Geometry: final body of the model. Coordinates: model frame, mm. Round coordinates to 2 decimals unless told otherwise and drop trailing zeros. Loops run counter-clockwise (first coordinate to the right, second up) from the corner with the lowest first, then second, coordinate; pieces in that order, holes last. Notation, with made-up numbers: (-18.75, 25.25) - (9.25, 25.25) arc R18 ccw to (9.25, 51.25) - close; hole circle Ø7 at (71.25, -12). An arc over 180 degrees is marked (long way). Return JSON: item names as keys, results as strings. Group by question number.
1. Section A-A on x = 0. Return loops of the section in (y, z), and give its area (3 significant figures).
2. Section B-B on y = -33.25. Return loops of the section in (x, z), and give its area (3 significant figures).
3. Section C-C on x = 84. Return loops of the section in (y, z).
4. First-contact query: pin 1 Ø5.5 at (x, y) = (-57.59, 33.25) entering from +Z. Flat tip, straight axial feed; report the tip coordinate or a pass-through.
5. Section D-D on z = 1.6. Count the separate pieces of the cut face and the enclosed holes in it, and give its area (3 significant figures).
6. Material intervals for probe 1 along Y at (x, z) = (47, 1.55); probe 2 along Y at (x, z) = (1, 2.45); probe 3 along X at (y, z) = (4, 1.3), sorted ascending.
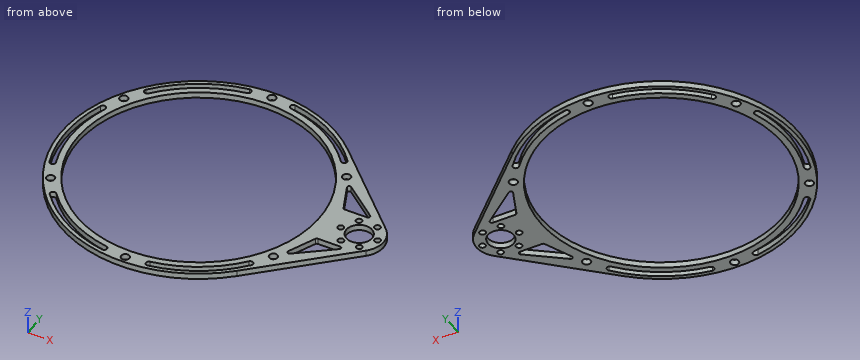
from build123d import *

# Parameters (mm, degrees)
SKETCH_1_R          = 2.1
SKETCH_1_R_2        = 61.75
SKETCH_1_R_3        = 1.55
SKETCH_1_R_4        = 6.6
EXTRUDE_1_DEPTH     = 3
CUT_EXTRUDE_1_DEPTH = 119.445134978
FILLET_1_R          = 1
CUT_EXTRUDE_2_DEPTH = 119.445134978


with BuildPart() as part:
    # 草图1 → 凸台-拉伸1 (new body)
    with BuildSketch(Plane.XY):
        with BuildLine():
            Line((91.659638554, 9.014469486), (48.493975904, 50.48102912))
            ThreePointArc((48.493975904, 50.48102912), (-70, 0), (48.493975904, -50.48102912))
            Line((48.493975904, -50.48102912), (91.659638554, -9.014469486))
            ThreePointArc((91.659638554, -9.014469486), (95.5, 0), (91.659638554, 9.014469486))
        make_face()
        with Locations((0, 66.5)):
            Circle(SKETCH_1_R, mode=Mode.SUBTRACT)
        with Locations((57.590689352, 33.25)):
            Circle(SKETCH_1_R, mode=Mode.SUBTRACT)
        with Locations((0, -66.5)):
            Circle(SKETCH_1_R, mode=Mode.SUBTRACT)
        with Locations((-57.590689352, -33.25)):
            Circle(SKETCH_1_R, mode=Mode.SUBTRACT)
        with Locations((57.590689352, -33.25)):
            Circle(SKETCH_1_R, mode=Mode.SUBTRACT)
        with Locations((-57.590689352, 33.25)):
            Circle(SKETCH_1_R, mode=Mode.SUBTRACT)
        Circle(SKETCH_1_R_2, mode=Mode.SUBTRACT)
        with Locations((87.75, 8.227241336)):
            Circle(SKETCH_1_R_3, mode=Mode.SUBTRACT)
        with Locations((78.25, -8.227241336)):
            Circle(SKETCH_1_R_3, mode=Mode.SUBTRACT)
        with Locations((87.75, -8.227241336)):
            Circle(SKETCH_1_R_3, mode=Mode.SUBTRACT)
        with Locations((73.5, 0)):
            Circle(SKETCH_1_R_3, mode=Mode.SUBTRACT)
        with Locations((83, 0)):
            Circle(SKETCH_1_R_4, mode=Mode.SUBTRACT)
        with Locations((78.25, 8.227241336)):
            Circle(SKETCH_1_R_3, mode=Mode.SUBTRACT)
        with Locations((92.5, 0)):
            Circle(SKETCH_1_R_3, mode=Mode.SUBTRACT)
    extrude(amount=EXTRUDE_1_DEPTH)

    # 草图2 → 切除-拉伸1 (cut, through all)
    with BuildSketch(Plane.XY.offset(3)):
        Polygon((59.859164826, 30.33893107), (67.889886949, 12.18949907), (83, 12.18949907), align=None)
        Polygon((67.889886949, -12.18949907), (83, -12.18949907), (59.859164826, -30.33893107), align=None)
    extrude(amount=-CUT_EXTRUDE_1_DEPTH, mode=Mode.SUBTRACT)

    # 圆角1
    fillet_1_edges = [part.edges().sort_by_distance(p)[0] for p in [
        (59.859164826, 30.33893107, 1.5),
        (83, 12.18949907, 1.5),
        (67.889886949, 12.18949907, 1.5),
        (59.859164826, -30.33893107, 1.5),
        (67.889886949, -12.18949907, 1.5),
        (83, -12.18949907, 1.5),
    ]]
    fillet(fillet_1_edges, radius=FILLET_1_R)

    # 草图3 → 切除-拉伸2 (cut, through all)
    with BuildSketch(Plane.XY.offset(3)):
        with BuildLine():
            ThreePointArc((52.091022132, 43.709557459), (34, 58.889727457), (11.808076081, 66.966927205))
            ThreePointArc((11.808076081, 66.966927205), (10.070392185, 65.750187842), (11.287131548, 64.012503946))
            ThreePointArc((11.287131548, 64.012503946), (32.5, 56.291651246), (49.792888803, 41.78119463))
            ThreePointArc((49.792888803, 41.78119463), (51.906136882, 41.596309379), (52.091022132, 43.709557459))
        make_face()
        with BuildLine():
            ThreePointArc((11.287131548, -64.012503946), (32.5, -56.291651246), (49.792888803, -41.78119463))
            ThreePointArc((49.792888803, -41.78119463), (51.906136882, -41.596309379), (52.091022132, -43.709557459))
            ThreePointArc((52.091022132, -43.709557459), (34, -58.889727457), (11.808076081, -66.966927205))
            ThreePointArc((11.808076081, -66.966927205), (10.070392185, -65.750187842), (11.287131548, -64.012503946))
        make_face()
        with BuildLine():
            ThreePointArc((-49.792888803, -41.78119463), (-32.5, -56.291651246), (-11.287131548, -64.012503946))
            ThreePointArc((-11.287131548, -64.012503946), (-10.070392185, -65.750187842), (-11.808076081, -66.966927205))
            ThreePointArc((-11.808076081, -66.966927205), (-34, -58.889727457), (-52.091022132, -43.709557459))
            ThreePointArc((-52.091022132, -43.709557459), (-51.906136882, -41.596309379), (-49.792888803, -41.78119463))
        make_face()
        with BuildLine():
            ThreePointArc((-61.080020351, 22.231309316), (-65, 0), (-61.080020351, -22.231309316))
            ThreePointArc((-61.080020351, -22.231309316), (-61.976529067, -24.153878462), (-63.899098213, -23.257369746))
            ThreePointArc((-63.899098213, -23.257369746), (-68, 0), (-63.899098213, 23.257369746))
            ThreePointArc((-63.899098213, 23.257369746), (-61.976529067, 24.153878462), (-61.080020351, 22.231309316))
        make_face()
        with BuildLine():
            ThreePointArc((-11.287131548, 64.012503946), (-32.5, 56.291651246), (-49.792888803, 41.78119463))
            ThreePointArc((-49.792888803, 41.78119463), (-51.906136882, 41.596309379), (-52.091022132, 43.709557459))
            ThreePointArc((-52.091022132, 43.709557459), (-34, 58.889727457), (-11.808076081, 66.966927205))
            ThreePointArc((-11.808076081, 66.966927205), (-10.070392185, 65.750187842), (-11.287131548, 64.012503946))
        make_face()
    extrude(amount=-CUT_EXTRUDE_2_DEPTH, mode=Mode.SUBTRACT)


solid = part.part
Taken from the geometry:
{
 "1": {"outline": "(-70, 0) - (-68.6, 0) - (-68.6, 3) - (-70, 3) - close; (-64.4, 0) - (-61.75, 0) - (-61.75, 3) - (-64.4, 3) - close; (61.75, 0) - (64.4, 0) - (64.4, 3) - (61.75, 3) - close; (68.6, 0) - (70, 0) - (70, 3) - (68.6, 3) - close", "area": "24.3 mm2"},
 "2": {"outline": "(-61.6, 0) - (-59.69, 0) - (-59.69, 3) - (-61.6, 3) - close; (-55.49, 0) - (-52.03, 0) - (-52.03, 3) - (-55.49, 3) - close; (52.03, 0) - (55.49, 0) - (55.49, 3) - (52.03, 3) - close; (59.69, 0) - (66.43, 0) - (66.43, 3) - (59.69, 3) - close", "area": "46.7 mm2"},
 "3": {"outline": "(-16.37, 0) - (-6.52, 0) - (-6.52, 3) - (-16.37, 3) - close; (6.52, 0) - (16.37, 0) - (16.37, 3) - (6.52, 3) - close"},
 "4": {"pin 1": "z = 3"},
 "5": {"separate pieces": "1", "enclosed holes": "21", "area": "3,270 mm2"},
 "6": {"probe 1": "-51.87 to -49.14, -44.9 to -40.05, 40.05 to 44.9, 49.14 to 51.87", "probe 2": "-69.99 to -68.35, -64.65 to -61.74, 61.74 to 64.65, 68.35 to 69.99", "probe 3": "-69.89 to -67.88, -64.88 to -61.62, 61.62 to 77.75, 88.25 to 94.84"}
}
